```python
from build123d import *

# Parameters (mm, degrees)
F1_DEPTH = 19.05
F2_R     = 5.08


with BuildPart() as f1:
    # F0 (on Top) → F1 (new body)
    with BuildSketch(Plane.XY):
        with BuildLine():
            Line((-353.695, 0), (-353.695, -154.782471149))
            ThreePointArc((-353.695, -154.782471149), (0, -386.08), (353.695, -154.782471149))
            Line((353.695, -154.782471149), (353.695, 0))
            Line((353.695, 0), (353.695, 154.782471149))
            ThreePointArc((353.695, 154.782471149), (0, 386.08), (-353.695, 154.782471149))
            Line((-353.695, 154.782471149), (-353.695, 0))
        make_face()
        with BuildLine():
            ThreePointArc((254.3058976541, 200.51766236), (305.9704131573, 106.1175233991), (323.85, 0))
            ThreePointArc((323.85, 0), (305.9704131573, -106.1175233991), (254.3058976541, -200.51766236))
            ThreePointArc((254.3058976541, -200.51766236), (255.9372994505, -255.9372994505), (200.51766236, -254.3058976541))
            ThreePointArc((200.51766236, -254.3058976541), (0, -323.85), (-200.51766236, -254.3058976541))
            ThreePointArc((-200.51766236, -254.3058976541), (-255.9372994505, -255.9372994505), (-254.3058976541, -200.51766236))
            ThreePointArc((-254.3058976541, -200.51766236), (-323.85, 0), (-254.3058976541, 200.51766236))
            ThreePointArc((-254.3058976541, 200.51766236), (-255.9372994505, 255.9372994505), (-200.51766236, 254.3058976541))
            ThreePointArc((-200.51766236, 254.3058976541), (0, 323.85), (200.51766236, 254.3058976541))
            ThreePointArc((200.51766236, 254.3058976541), (255.9372994505, 255.9372994505), (254.3058976541, 200.51766236))
        make_face(mode=Mode.SUBTRACT)
    extrude(amount=F1_DEPTH)

    # F2
    f2_edges = [f1.edges().sort_by_distance(p)[0] for p in [
        (0, 323.85, 19.05),
        (323.85, 0, 19.05),
        (0, 323.85, 0),
        (323.85, 0, 0),
        (0, -323.85, 19.05),
        (-323.85, 0, 19.05),
        (-323.85, 0, 0),
        (0, -323.85, 0),
    ]]
    fillet(f2_edges, radius=F2_R)


solid = f1.part
```
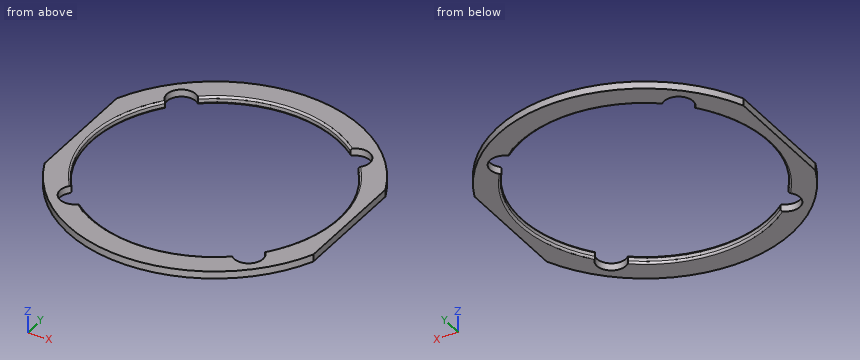
The listing builds one solid part. Answer for the finished solid, in the listing's coordinates (mm). Coordinates: 2 decimals unless noted, no trailing zeros. Order: outer loops, then holes, each group sorted by start corner. A loop starts at its lowest first (then second) coordinate and runs counter-clockwise, first axis right, second up. Notation, with made-up numbers: M -34,-39.75 L -2,-39.75 A30 cw -2,-7.75 Z; hole C -13.75,19 d8. An arc over 180 degrees is marked long. Answer as a JSON object with one key per item and string values. Group by question number.
1. Straight lines are drawn through the part: line 1 (X direction, y = 15, z = 16) (3 decimals); line 2 (X direction, y = -18, z = 16.5) (3 decimals); line 3 (Y direction, x = -4, z = 8). For each, find the intervals that lie inside material, in ascending order.
2. Flat-ended cylindrical pins translate along their axes: P1, Ø2, axis at y = -200.5, z = 16.5, coming from the +X side; P2, Ø10, axis at x = 69.5, z = 15, coming from the +Y side; P3, Ø10, axis at x = -70, z = 3.5, coming from the +Y side. Find the tip coordinate at first contact, or state that the pin passes through.
3. Section A-A on z = 10 is taken. Write down the section's boundary in (x, y) (3 decimals).
Values follow:
{
 "1": {"line 1": "-353.695 to -323.926, 323.926 to 353.695", "line 2": "-353.695 to -324.025, 324.025 to 353.695", "line 3": "-386.06 to -323.83, 323.83 to 386.06"},
 "2": {"P1": "x = 330.54", "P2": "y = 380.65", "P3": "y = 380.57"},
 "3": {"outline": "M -353.695,-154.782 A386.08 ccw 353.695,-154.782 L 353.695,154.782 A386.08 ccw -353.695,154.782 Z; hole M -254.306,-200.518 A38.1 ccw long -200.518,-254.306 A323.85 ccw 200.518,-254.306 A38.1 ccw long 254.306,-200.518 A323.85 ccw 254.306,200.518 A38.1 ccw long 200.518,254.306 A323.85 ccw -200.518,254.306 A38.1 ccw long -254.306,200.518 A323.85 ccw Z"}
}
